Input: part model. Units: mm. Frame: model coordinates. Round coordinates to 2 decimals unless told otherwise and drop trailing zeros. Loops run counter-clockwise (first coordinate to the right, second up) from the corner with the lowest first, then second, coordinate; pieces in that order, holes last.
1) Section A-A, the plane y = 1.65. Return loops of the section in (x, z), and give its area (3 significant figures).
2) Ray query, line 1 along X through (y, z) = (0.85, 14.8); line 2 along X through (y, z) = (1.7, -10); line 3 along Z through (x, y) = (-39.5, 2.1). Return the intervals inside material, ascending.
3) First-contact query: pin 1 (0.9 mm diameter, centred on x = -23.5, y = 1.5, fed in from -Z); pin 2 (1.2 mm diameter, centred on y = 1, z = -7.5, fed in from +X); pin 3 (2 mm diameter, centred on x = -81.406, z = -125, fed in from -Y); pin 4 (1.2 mm diameter, centred on x = -98.5, y = 1.5, fed in from +Z). Flat tips, straight axial feed; report the tip coordinate or a pass-through.
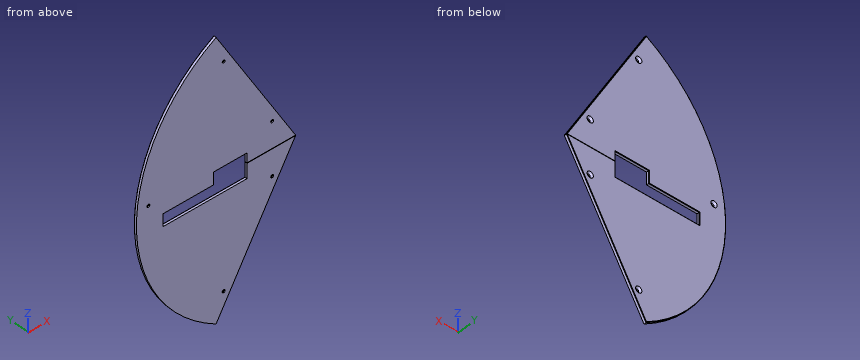
Autodesk Inventor part; units mm, degrees
ref_plane "YZ Plane" through (0, 0, 0) normal (1, 0, 0) x (0, 1, 0)
ref_plane "XZ Plane" through (0, 0, 0) normal (0, 1, 0) x (-1, 0, 0)
ref_plane "XY Plane" through (0, 0, 0) normal (0, 0, 1) x (1, 0, 0)
sketch "Skizze1" plane through (0, 0, 0) normal (0, 1, 0) x (-1, 0, 0)
  line L0 (0, 0) -> (90, 155.8846)
  line L1 (0, 0) -> (90, -155.8846)
  arc A0 (90, -155.8846) -> (90, 155.8846) centre (0, 0) ccw
  line L2 (216, 0) -> (-36, 0)
  dimension "d0" = 360
  dimension "d1" = 120
  dimension "d2" = 60
extrude "Extrusion1" add sketch "Skizze1" along normal blind 3
fillet "Rundung1" radius 0.5 3 edges at (-45, 3, 77.9423) (-180, 3, 0) (-45, 3, -77.9423)
sketch "Skizze2" plane through (0, 3, 0) normal (0, 1, 0) x (1, 0, 0)
  line L0 (-150, 3) -> (-93, 3)
  line L1 (-55, 3) -> (-55, 17)
  line L2 (-55, 17) -> (-150, 17)
  line L3 (-150, 17) -> (-150, 3)
  line L4 (-227.898, 0) -> (107.3877, 0)
  line L5 (-93, 3) -> (-93, -11)
  line L6 (-93, -11) -> (-55, -11)
  line L7 (-55, -11) -> (-55, 3)
  point P0 (0, 0)
  point P1 (-55, 10)
  point P2 (-150, 10)
  dimension "d6" = 14
  dimension "d7" = 95
  dimension "d8" = 17
  dimension "d10" = 150
  dimension "d13" = 38
  dimension "d14" = 14
extrude "Extrusion2" cut sketch "Skizze2" against normal blind 3
fillet "Rundung2" radius 0.5 6 edges at (-102.5, 3, -17) (-121.5, 3, -3) (-150, 3, -10) (-93, 3, 4) (-74, 3, 11) (-55, 3, -3)
sketch "Skizze3" plane through (0, 3, 0) normal (0, 1, 0) x (1, 0, 0)
  line L0 (0, -0.25) -> (-60, -0.25)
  line L1 (-60, -0.25) -> (-60, 0.25)
  line L2 (-60, 0.25) -> (0, 0.25)
  line L3 (0, 0.25) -> (0, -0.25)
  line L4 (-216, 0) -> (36, 0)
  point P0 (0, 0)
  point P1 (0, 0)
  dimension "d16" = 0.5
  dimension "d17" = 0.25
  dimension "d18" = 60
  dimension "d19" = 0
extrude "Extrusion3" cut sketch "Skizze3" against normal blind 3
sketch "Skizze4" plane through (0, 3, 0) normal (0, 1, 0) x (1, 0, 0)
  circle A0 centre (-81.406, -125) radius 1.65
  circle A1 centre (-26.558, -30) radius 1.65
  circle A2 centre (-166.5, -14.8) radius 1.65
  circle A3 centre (-81.406, 125) radius 1.65
  circle A4 centre (-26.558, 30) radius 1.65
  point P0 (0, 0)
  dimension "d26" = 26.558
  dimension "d27" = 26.558
  dimension "d28" = 3.3
  dimension "d29" = 81.406
  dimension "d30" = 81.406
  dimension "d31" = 14.8
  dimension "d32" = 166.5
  dimension "d33" = 125
  dimension "d34" = 30
  dimension "d35" = 30
  dimension "d36" = 125
extrude "Extrusion4" cut sketch "Skizze4" against normal blind 3
chamfer "Fasen1" distance 1.9 angle 45 5 edges at (-83.056, 3, -125) (-28.208, 3, -30) (-28.208, 3, 30) (-83.056, 3, 125) (-168.15, 3, 14.8)
properties part number "cover"
Final values:
1. outline: (-150, -17) - (-150, -3) - (-93, -3) - (-93, 11) - (-55, 11) - (-55, 0.25) - (-0.14, 0.25) - (-90, 155.88) arc R180 ccw to (-90, -155.88) - (-0.14, -0.25) - (-55, -0.25) - (-55, -17) - close; hole circle Ø4.4 at (-166.5, 14.8); hole circle Ø4.4 at (-81.41, -125); hole circle Ø4.4 at (-81.41, 125); hole circle Ø4.4 at (-26.56, -30); hole circle Ø4.4 at (-26.56, 30)
1. area: 32,000 mm2
2. line 1: x = -179.39 to -168.15, -164.85 to -8.54
2. line 2: x = -179.72 to -150, -55 to -5.77
2. line 3: z = -68.42 to -0.25, 0.25 to 68.42
3. pin 1: stops at z = -41.48
3. pin 2: stops at x = -3.98
3. pin 3: passes through
3. pin 4: stops at z = 151.05
